Verification items for this drawing (mm, ordinates from the low corner). A direction names the side the tool comes from. Coordinates: 2 decimals unless noted, no trailing zeros. Write each loop counter-clockwise with the first axis right and the second up, starting at its lowest first coordinate (ties: lowest second). Pieces come first, ordered by that corner, then holes.
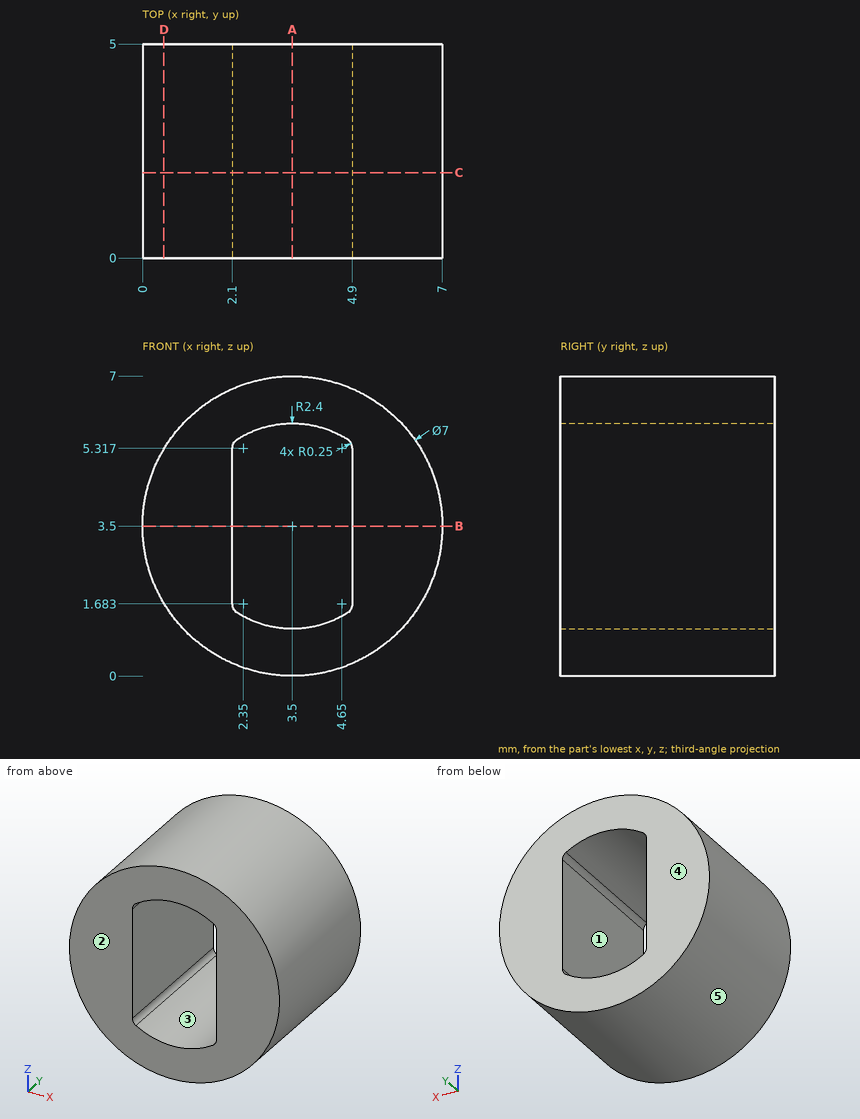
1. Gauge pin test, flat end, axial feed: pin 1 Ø1.5 at (x, y) = (4.5, 1) entering from +Z. Record the tip position at first contact, or that the pin passes through.
Computed values:
pin 1: stops at z = 6.99
2. Sectioned sample at A-A, the plane x = 3.5. Record the boundary of the cut face in (y, z), and give its area (3 significant figures).
Computed values:
outline: (0, 0) - (5, 0) - (5, 1.1) - (0, 1.1) - close; (0, 5.9) - (5, 5.9) - (5, 7) - (0, 7) - close
area: 11.0 mm2
3. Sectioned sample at B-B, the plane z = 3.5. Record the boundary of the cut face in (x, y), and give its area (3 significant figures).
Computed values:
outline: (0, 0) - (2.1, 0) - (2.1, 5) - (0, 5) - close; (4.9, 0) - (7, 0) - (7, 5) - (4.9, 5) - close
area: 21.0 mm2
4. Draft check along Z on the marked faces 3, 4 and 5. Enter one of: released by +Z, released by -Z, zero draft, split by the parting line, or undercut.
Computed values:
face 3: undercut
face 4: zero draft
face 5: split by the parting line
5. Thickness scan on line 1 along X through (y, z) = (4.3, 1.5) (1 decimal); line 2 along X through (y, z) = (1.85, 4.75); line 3 along Z through (x, y) = (4.25, 4). Record the ranges inside material, lowest first.
Computed values:
line 1: x = 0.6 to 2.2, 4.8 to 6.4
line 2: x = 0.23 to 2.1, 4.9 to 6.77
line 3: z = 0.08 to 1.22, 5.78 to 6.92
6. Access from +Z, -Z, +X, -X, +Y, -Y to the whole of each face (thin tool, end or side, straight path). Record for the marked faces 1 and 2.
Computed values:
face 1: +Y, -Y
face 2: +Z, -Z, +X, -X, -Y
7. Sectioned sample at C-C, the plane y = 2. Record the boundary of the cut face in (x, z).
Computed values:
outline: circle Ø7 at (3.5, 3.5); hole (2.1, 1.68) arc R0.25 ccw to (2.22, 1.47) arc R2.4 ccw to (4.78, 1.47) arc R0.25 ccw to (4.9, 1.68) - (4.9, 5.32) arc R0.25 ccw to (4.78, 5.53) arc R2.4 ccw to (2.22, 5.53) arc R0.25 ccw to (2.1, 5.32) - close
8. Sectioned sample at D-D, the plane x = 0.5. Record the boundary of the cut face in (y, z), and give its area (3 significant figures).
Computed values:
outline: (0, 1.7) - (5, 1.7) - (5, 5.3) - (0, 5.3) - close
area: 18.0 mm2
